from build123d import *

# Parameters (mm, degrees)
SKETCH1_R           = 3.95
SKETCH1_R_2         = 1.475
SKETCH1_R_3         = 13.5
SKETCH1_R_4         = 2.5
BOSS_EXTRUDE1_DEPTH = 5


with BuildPart() as part:
    # Sketch1 → Boss-Extrude1 (new body)
    with BuildSketch(Plane.XY):
        with BuildLine():
            Line((35, 0), (35, 162))
            ThreePointArc((35, 162), (0, 197), (-35, 162))
            Line((-35, 162), (-35, 0))
            ThreePointArc((-35, 0), (0, -35), (35, 0))
        make_face()
        Circle(SKETCH1_R, mode=Mode.SUBTRACT)
        with Locations((15.5, 15.5)):
            Circle(SKETCH1_R_2, mode=Mode.SUBTRACT)
        with Locations((15.5, -15.5)):
            Circle(SKETCH1_R_2, mode=Mode.SUBTRACT)
        with Locations((-15.5, -15.5)):
            Circle(SKETCH1_R_2, mode=Mode.SUBTRACT)
        with Locations((-15.5, 15.5)):
            Circle(SKETCH1_R_2, mode=Mode.SUBTRACT)
        with Locations((0, 29)):
            Circle(SKETCH1_R_2, mode=Mode.SUBTRACT)
        with Locations((0, 162)):
            Circle(SKETCH1_R_3, mode=Mode.SUBTRACT)
        with Locations((-18, 162)):
            Circle(SKETCH1_R_4, mode=Mode.SUBTRACT)
        with Locations((18, 162)):
            Circle(SKETCH1_R_4, mode=Mode.SUBTRACT)
        with Locations((0, 133)):
            Circle(SKETCH1_R_2, mode=Mode.SUBTRACT)
        with Locations((-30, 97)):
            Circle(SKETCH1_R_2, mode=Mode.SUBTRACT)
        with Locations((30, 97)):
            Circle(SKETCH1_R_2, mode=Mode.SUBTRACT)
        with Locations((29, 0)):
            Circle(SKETCH1_R_2, mode=Mode.SUBTRACT)
        with Locations((0, -29)):
            Circle(SKETCH1_R_2, mode=Mode.SUBTRACT)
        with Locations((-29, 0)):
            Circle(SKETCH1_R_2, mode=Mode.SUBTRACT)
        with BuildLine():
            Line((2.4, 54.5), (2.4, 39.5))
            ThreePointArc((2.4, 39.5), (0, 37.1), (-2.4, 39.5))
            Line((-2.4, 39.5), (-2.4, 54.5))
            ThreePointArc((-2.4, 54.5), (0, 56.9), (2.4, 54.5))
        make_face(mode=Mode.SUBTRACT)
        with BuildLine():
            Line((2.4, 80.5), (2.4, 65.5))
            ThreePointArc((2.4, 65.5), (0, 63.1), (-2.4, 65.5))
            Line((-2.4, 65.5), (-2.4, 80.5))
            ThreePointArc((-2.4, 80.5), (0, 82.9), (2.4, 80.5))
        make_face(mode=Mode.SUBTRACT)
        with BuildLine():
            Line((19.4, 67.5), (19.4, 52.5))
            ThreePointArc((19.4, 52.5), (17, 50.1), (14.6, 52.5))
            Line((14.6, 52.5), (14.6, 67.5))
            ThreePointArc((14.6, 67.5), (17, 69.9), (19.4, 67.5))
        make_face(mode=Mode.SUBTRACT)
        with BuildLine():
            Line((-19.4, 67.5), (-19.4, 52.5))
            ThreePointArc((-19.4, 52.5), (-17, 50.1), (-14.6, 52.5))
            Line((-14.6, 52.5), (-14.6, 67.5))
            ThreePointArc((-14.6, 67.5), (-17, 69.9), (-19.4, 67.5))
        make_face(mode=Mode.SUBTRACT)
        with BuildLine():
            Line((6.5, 121.5), (6.5, 108.5))
            ThreePointArc((6.5, 108.5), (0, 102), (-6.5, 108.5))
            Line((-6.5, 108.5), (-6.5, 121.5))
            ThreePointArc((-6.5, 121.5), (0, 128), (6.5, 121.5))
        make_face(mode=Mode.SUBTRACT)
        with BuildLine():
            Line((26.5, 120.946496324), (26.5, 107.946496324))
            ThreePointArc((26.5, 107.946496324), (20, 101.446496324), (13.5, 107.946496324))
            Line((13.5, 107.946496324), (13.5, 120.946496324))
            ThreePointArc((13.5, 120.946496324), (20, 127.446496324), (26.5, 120.946496324))
        make_face(mode=Mode.SUBTRACT)
        with BuildLine():
            Line((-26.5, 120.946496324), (-26.5, 107.946496324))
            ThreePointArc((-26.5, 107.946496324), (-20, 101.446496324), (-13.5, 107.946496324))
            Line((-13.5, 107.946496324), (-13.5, 120.946496324))
            ThreePointArc((-13.5, 120.946496324), (-20, 127.446496324), (-26.5, 120.946496324))
        make_face(mode=Mode.SUBTRACT)
    extrude(amount=BOSS_EXTRUDE1_DEPTH)


solid = part.part
Part model, mm, in its own coordinate system. A direction names the side the tool comes from. Round coordinates to 2 decimals unless told otherwise and drop trailing zeros. Write each loop counter-clockwise with the first axis right and the second up, starting at its lowest first coordinate (ties: lowest second). Pieces come first, ordered by that corner, then holes. Notation, with made-up numbers: M 21,0.25 L 78,0.25 A26 cw 78,15.25 Z; hole C 38.5,40.5 d11. An arc over 180 degrees is marked long. Return JSON: item names as keys, results as strings. Group by question number.
(1) Saw through at A-A on y = 76.5. Write the cut outline in (x, z), then the cut area to 3 significant figures.
(2) Two-plate mould, pull along X, no slides. Class faces 3 (the face through (7, 83, 0)), 4 (the face through (-26.5, 115, 2)), 5 (the face through (-0.77, -34.99, 2.46)): +X half, -X half, draft (parallel to the pull), parting line (faces both ways), or undercut.
(3) Which spindle directions (+Z, -Z, +X, -X, +Y, -Y) get a long thin tool onto all of the face, cutting with end or side? Do faces 1 (the face through (-19.4, 60, 2)), 2 (the face through (0.77, 196.99, 2.46)). Say none if no direction does.
(4) Saw through at D-D on y = 178. Write the cut outline in (x, z).
(5) Saw through at B-B on x = 22.5. Write the cut outline in (y, z).
(6) Saw through at C-C on z = 3.1. Count the separate pieces of the cut face and the enclosed holes in it, then the cut area to 3 significant figures.
(7) Drill centre lines: probe 1 along X at (y, z) = (97, 3.5) (3 decimals); probe 2 along X at (y, z) = (59, 1.3); probe 3 along X at (y, z) = (107.5, 1.3). Where is each one in solid material? Low to high.
(8) Pin check, flat tip, straight feed: pin 1 Ø1 at (x, z) = (-12, 2.5) entering from +Y. Stop position of the tip, or through.
Returned:
{
 "1": {"outline": "M -35,0 L -2.4,0 L -2.4,5 L -35,5 Z; M 2.4,0 L 35,0 L 35,5 L 2.4,5 Z", "area": "326 mm²"},
 "2": {"face 3": "draft", "face 4": "undercut", "face 5": "parting line"},
 "3": {"face 1": "+Z, -Z", "face 2": "+Z, -Z, +Y"},
 "4": {"outline": "M -31.13,0 L 31.13,0 L 31.13,5 L -31.13,5 Z"},
 "5": {"outline": "M -26.81,0 L 101.95,0 L 101.95,5 L -26.81,5 Z; M 126.95,0 L 188.81,0 L 188.81,5 L 126.95,5 Z"},
 "6": {"separate pieces": "1", "enclosed holes": "22", "area": "13,200 mm²"},
 "7": {"probe 1": "-35 to -31.475, -28.525 to 28.525, 31.475 to 35", "probe 2": "-35 to -19.4, -14.6 to 14.6, 19.4 to 35", "probe 3": "-35 to -26.48, -13.52 to -6.42, 6.42 to 13.52, 26.48 to 35"},
 "8": {"pin 1": "y = 195.06"}
}
